Can you work these out from the model? Positions are in its coordinate system, mm. A direction names the side the tool comes from. Coordinates: 2 decimals unless noted, no trailing zeros. Order: outer loops, then holes, each group sorted by start corner. A loop starts at its lowest first (then second) coordinate and runs counter-clockwise, first axis right, second up. Notation, with made-up numbers: (40, 75) -> (79, 75) arc R6 ccw to (79, 85) -> close; hole circle Ø11 at (5.5, -39.75). An arc over 180 degrees is marked (long way). Return JSON: item names as keys, results as strings. Group by question number.
1) For pin 1 (4 mm diameter, centred on y = 0, z = 227.457, fed in from +X), with a flat end and sliding along its axis, tell me the tip position at first contact or that it passes through.
2) For faces 5 (the flat face through (15.875, 0, -4)), 6 (the flat face through (0, -11, 317.5)), which set-ups out of +Z, -Z, +X, -X, +Y, -Y let a thin tool reach every point of the face, with its end or its side?
3) If I drill on probe 1 along Z at (x, y) = (12.7, 11.85); probe 2 along Y at (x, z) = (-14, 55) (3 decimals); probe 3 along Y at (x, z) = (-17, -279), over which ranges is the centre line in solid material (lowest first)? Write a range as from..to.
4) Thinking about a two-plate mould opening in Z: for faces 1 (the flat face through (0, -11, -317.5)), 2 (the conical face through (-13.49, -9.71, 27.9)), 3 (the conical face through (14.295, -9.711, -27.481)), 4 (the flat face through (0, -9.525, -4)), which applies, +Z half, -Z half, draft (parallel to the pull), parting line (faces both ways), or undercut?
5) If we section it at A-A, the plane z = 70: Please give me the cut outline in (x, y) (3 decimals).
6) If we section it at B-B, the plane x = -2: Please give me the cut outline in (y, z) (3 decimals).
from build123d import *

# Parameters (mm, degrees)
BOSS_EXTRUDE1_DEPTH             = 317.499999
BOSS_EXTRUDE1_DEPTH_BACK        = 317.499999
SKETCH3_W                       = 38.1
SKETCH3_H                       = 25.4
SKETCH3_W_2                     = 31.75
SKETCH3_H_2                     = 19.05
F_10_CLEARANCE_HOLE2_D          = 4.9784
F_10_CLEARANCE_HOLE5_D          = 4.9784
F_10_CLEARANCE_HOLE4_D          = 4.9784
F_10_CLEARANCE_HOLE3_D          = 4.9784
F_10_CLEARANCE_HOLE6_AT_2_COUNT = 2
F_10_CLEARANCE_HOLE6_AT_2_PITCH = 25.4
F_10_CLEARANCE_HOLE6_AT_3_COUNT = 2
F_10_CLEARANCE_HOLE6_AT_3_PITCH = 50.8
F_10_CLEARANCE_HOLE6_AT_4_COUNT = 2
F_10_CLEARANCE_HOLE6_AT_4_PITCH = 56.796126628
F_10_CLEARANCE_HOLE7_D          = 4.9784


with BuildPart() as part:
    # Sketch3 → Boss-Extrude1 (new, two sides: drawn at the far end of the back side and taken through both)
    with BuildSketch(Plane.XY.offset(-BOSS_EXTRUDE1_DEPTH_BACK)):
        Rectangle(SKETCH3_W, SKETCH3_H)
        Rectangle(SKETCH3_W_2, SKETCH3_H_2, mode=Mode.SUBTRACT)
    extrude(amount=BOSS_EXTRUDE1_DEPTH + BOSS_EXTRUDE1_DEPTH_BACK)

    # #10 Clearance Hole2 (through all)
    with Locations(Plane.ZY.offset(19.05)):
        with Locations((-304.799999492, 0), (-279.399999492, 0), (279.400000508, 0), (304.800000508, 0)):
            Hole(F_10_CLEARANCE_HOLE2_D / 2)

    # #10 Clearance Hole5 (through all)
    with Locations(Plane(origin=(19.05, 0, 0), x_dir=(0, 0, -1), z_dir=(1, 0, 0))):
        with Locations((-124.587000508, -1.231595708), (-99.187000508, -1.231595708), (-252.857000508, -5.03e-07), (-227.457000508, -5.03e-07)):
            Hole(F_10_CLEARANCE_HOLE5_D / 2)

    # #10 Clearance Hole4 (through all)
    with Locations(Plane(origin=(19.05, 0, 0), x_dir=(0, 0, -1), z_dir=(1, 0, 0))):
        with Locations((-252.857000508, -5.03e-07), (-227.457000508, -5.03e-07)):
            Hole(F_10_CLEARANCE_HOLE4_D / 2)

    # #10 Clearance Hole3 (through all)
    with Locations(Plane.ZY.offset(19.05)):
        with Locations((-50.8, 0), (50.8, 0)):
            Hole(F_10_CLEARANCE_HOLE3_D / 2)

    # Sketch26 → #10 Clearance Hole6 (revolve, cut)
    with BuildSketch(Plane(origin=(12.7, 12.7, 25.4), x_dir=(0, 0, 1), z_dir=(1, 0, 0))):
        Polygon((0, 0), (0, 25.4), (5.2197, 25.4), (2.4892, 22.258919064), (2.4892, 0), align=None)
    f_10_clearance_hole6 = revolve(axis=Axis((12.7, 19.05, 25.4), (0, -1, 0)), mode=Mode.SUBTRACT)

    # #10 Clearance Hole6 at 2: #10 Clearance Hole6 ×2
    with Locations(*[(-i * F_10_CLEARANCE_HOLE6_AT_2_PITCH, 0, 0) for i in range(1, F_10_CLEARANCE_HOLE6_AT_2_COUNT)]):
        add(f_10_clearance_hole6, mode=Mode.SUBTRACT)

    # #10 Clearance Hole6 at 3: #10 Clearance Hole6 ×2
    with Locations(*[(0, 0, -i * F_10_CLEARANCE_HOLE6_AT_3_PITCH) for i in range(1, F_10_CLEARANCE_HOLE6_AT_3_COUNT)]):
        add(f_10_clearance_hole6, mode=Mode.SUBTRACT)

    # #10 Clearance Hole6 at 4: #10 Clearance Hole6 ×2
    with Locations(*[Vector(-0.447213595499958, 0, -0.894427190999916) * (i * F_10_CLEARANCE_HOLE6_AT_4_PITCH) for i in range(1, F_10_CLEARANCE_HOLE6_AT_4_COUNT)]):
        add(f_10_clearance_hole6, mode=Mode.SUBTRACT)

    # #10 Clearance Hole7 (through all)
    with Locations(Plane.ZY.offset(19.05)):
        with Locations((-95.25, 0)):
            Hole(F_10_CLEARANCE_HOLE7_D / 2)


solid = part.part
Result sheet:
{
 "1": {"pin 1": "passes through"},
 "2": {"face 5": "+Z, -Z", "face 6": "+Z, +X, -X, +Y, -Y"},
 "3": {"probe 1": "z = -317.5..-27.89, -22.91..22.91, 27.89..317.5", "probe 2": "y = -12.7..-9.525, 9.525..12.7", "probe 3": "y = -12.7..-2.46, 2.46..12.7"},
 "4": {"face 1": "-Z half", "face 2": "undercut", "face 3": "undercut", "face 4": "draft"},
 "5": {"outline": "(-19.05, -12.7) -> (19.05, -12.7) -> (19.05, 12.7) -> (-19.05, 12.7) -> close; hole (-15.875, -9.525) -> (15.875, -9.525) -> (15.875, 9.525) -> (-15.875, 9.525) -> close"},
 "6": {"outline": "(-12.7, -317.5) -> (-9.525, -317.5) -> (-9.525, 317.5) -> (-12.7, 317.5) -> close; (9.525, -317.5) -> (12.7, -317.5) -> (12.7, 317.5) -> (9.525, 317.5) -> close"}
}
